CAD build for the part. Positions are in the model's coordinates, mm. Face numbers are marked on the shaded views. A direction names the side the tool comes from. Round coordinates to 2 decimals unless told otherwise and drop trailing zeros. Loops run counter-clockwise (first coordinate to the right, second up) from the corner with the lowest first, then second, coordinate; pieces in that order, holes last. Notation, with made-up numbers: M -14.75,4.5 L -2.75,4.5 A18 ccw -2.75,19.5 Z; hole C 67,85 d6. An arc over 180 degrees is marked long. Use a Markdown table: item, result. Add a question column.
(1) Band-saw the part on D-D, the plane y = 2. Write the cut outline in (x, z) (3 decimals), and give its area (3 significant figures).
(2) Band-saw the part on B-B, the plane x = 10.5. Write the cut outline in (y, z).
(3) Two-plate mould, pull along X, no slides. Class the marked faces 3, 4 and 5: released by +X, released by -X, zero draft, split by the parting line, or undercut.
(4) Wall check: L1, parallel to Z at x = 36.9, y = 12.7; L2, parallel to X at y = 27, z = 12.5; L3, parallel to Z at x = 37.85, y = 12.7. Give the ranges that are in metal, low to high.
(5) Band-saw the part on C-C, the plane z = 21.5. Write the cut outline in (x, y), and give its area (3 significant figures).
(6) Flat gauge pins, fed straight in: P1, Ø5.5, axis at y = 12.7, z = 66.075, coming from the -X side; P2, Ø6, axis at x = -15, z = 7.5, coming from the -Y side; P3, Ø3.5, axis at x = -14.5, y = 20.5, coming from the +Z side; P4, Ø7.5, axis at y = 25, z = 11, coming from the -X side. Where does each tip first touch, or does it go through?
(7) Band-saw the part on A-A, the plane y = 12.7. Give the number of separate pieces and of enclosed holes in the cut face, and give its area (3 significant figures).
(8) Which spindle directions (+Z, -Z, +X, -X, +Y, -Y) get a long thin tool onto all of the face, cutting with end or side? Do the marked faces 1 and 2. Say none if no direction does.
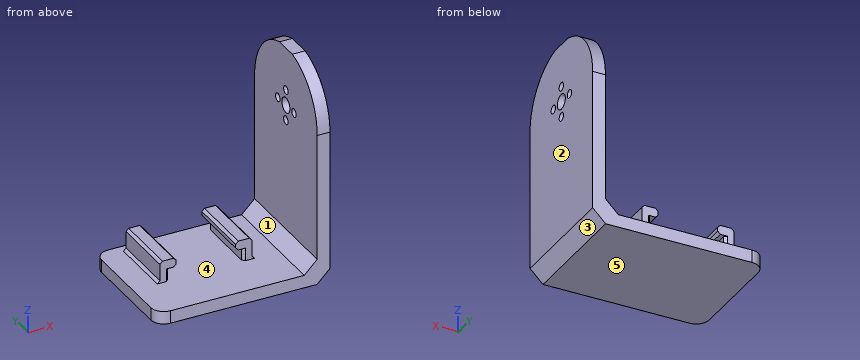
from build123d import *

# Parameters (mm, degrees)
F0_W      = 57.15
F0_H      = 21.6
F1_DEPTH  = 5
F2_W      = 57.15
F2_H      = 25.4
F3_DEPTH  = 5
F4_W      = 3.556
F4_H      = 25.4
F5_DEPTH  = 5.08
F6_W      = 6.35
F6_H      = 25.4
F7_DEPTH  = 3.556
F8_SIZE   = 1.016
F9_W      = 10.425
F9_H      = 47
F10_DEPTH = 5
F11_W     = 5
F11_H     = 47
F12_DEPTH = 78
F13_R     = 1.6478
F13_R_2   = 3
F14_DEPTH = 25.4
F16_DEPTH = 25.4
F17_R     = 5.08
F18_SIZE  = 5.08


with BuildPart() as f1:
    # F0 (on Top) → F1 (new body)
    with BuildSketch(Plane.XY):
        Rectangle(F0_W, F0_H)
    extrude(amount=F1_DEPTH)

    # F2 (on Top) → F3 (join)
    with BuildSketch(Plane.XY):
        with Locations((0, 23.5)):
            Rectangle(F2_W, F2_H)
    extrude(amount=F3_DEPTH)

    # F4 (on face) → F5 (join)
    with BuildSketch(Plane.XY.offset(5)):
        with Locations((-16.256, 20.32)):
            Rectangle(F4_W, F4_H)
        with Locations((16.256, 20.32)):
            Rectangle(F4_W, F4_H)
    extrude(amount=F5_DEPTH)

    # F6 (on face) → F7 (join)
    with BuildSketch(Plane.XY.offset(10.08)):
        with Locations((-14.859, 20.32)):
            Rectangle(F6_W, F6_H)
        with Locations((14.859, 20.32)):
            Rectangle(F6_W, F6_H)
    extrude(amount=F7_DEPTH)

    # F8
    f8_edges = [f1.edges().sort_by_distance(p)[0] for p in [
        (-11.684, 20.32, 13.636),
        (-11.684, 20.32, 10.08),
        (11.684, 20.32, 13.636),
        (11.684, 20.32, 10.08),
        (18.034, 20.32, 13.636),
        (-18.034, 20.32, 13.636),
        (18.034, 20.32, 5),
        (-18.034, 20.32, 5),
        (14.478, 33.02, 7.54),
        (-14.478, 33.02, 7.54),
        (-14.478, 7.62, 7.54),
        (14.478, 7.62, 7.54),
    ]]
    chamfer(f8_edges, length=F8_SIZE)

    # F9 (on face) → F10 (join)
    with BuildSketch(Plane.XY.offset(5)):
        with Locations((33.7875, 12.7)):
            Rectangle(F9_W, F9_H)
    extrude(amount=-F10_DEPTH)

    # F11 (on face) → F12 (join)
    with BuildSketch(Plane.XY.offset(5)):
        with Locations((36.5, 12.7)):
            Rectangle(F11_W, F11_H)
    extrude(amount=F12_DEPTH)

    # F13 (on face) → F14 (cut)
    with BuildSketch(Plane.YZ.offset(39)):
        with Locations((6.625, 60)):
            Circle(F13_R)
        with Locations((12.7, 53.925)):
            Circle(F13_R)
        with Locations((18.775, 60)):
            Circle(F13_R)
        with Locations((12.7, 66.075)):
            Circle(F13_R)
        with Locations((12.7, 60)):
            Circle(F13_R_2)
    extrude(amount=-F14_DEPTH, mode=Mode.SUBTRACT)

    # F15 (on face) → F16 (cut)
    with BuildSketch(Plane(origin=(34, 0, 0), x_dir=(0, -1, 0), z_dir=(-1, 0, 0))):
        with BuildLine():
            ThreePointArc((-36.2, 60), (-30.942298, 74.814471), (-17.521825, 83))
            Line((-17.521825, 83), (-36.2, 83))
            Line((-36.2, 83), (-36.2, 60))
        make_face()
        with BuildLine():
            Line((-17.521825, 83), (-7.878175, 83))
            ThreePointArc((-7.878175, 83), (-12.7, 83.5), (-17.521825, 83))
        make_face()
        with BuildLine():
            ThreePointArc((-7.878175, 83), (5.542298, 74.814471), (10.8, 60))
            Line((10.8, 60), (10.8, 83))
            Line((10.8, 83), (-7.878175, 83))
        make_face()
    extrude(amount=-F16_DEPTH, mode=Mode.SUBTRACT)

    # F17
    f17_edges = [f1.edges().sort_by_distance(p)[0] for p in [
        (-28.575, -10.8, 2.5),
        (-28.575, 36.2, 2.5),
    ]]
    fillet(f17_edges, radius=F17_R)

    # F18
    f18_edges = [f1.edges().sort_by_distance(p)[0] for p in [
        (34, 12.7, 5),
        (39, 12.7, 0),
    ]]
    chamfer(f18_edges, length=F18_SIZE)


solid = f1.part
Return value:
| question | item | result |
|---|---|---|
| 1 | outline | M -28.575,0 L 33.92,0 L 39,5.08 L 39,80.923 L 34,80.923 L 34,10.08 L 28.92,5 L -28.575,5 Z |
| 1 | area | 717 mm^2 |
| 2 | outline | M -10.8,0 L 36.2,0 L 36.2,5 L -10.8,5 Z |
| 3 | face 3 | released by +X |
| 3 | face 4 | undercut |
| 3 | face 5 | zero draft |
| 4 | L1 | 2.98 to 52.28, 55.57 to 57, 63 to 64.43, 67.72 to 83 |
| 4 | L2 | -18.03 to -11.68, 11.68 to 18.03, 34 to 39 |
| 4 | L3 | 3.93 to 52.28, 55.57 to 57, 63 to 64.43, 67.72 to 83 |
| 5 | outline | M 34,-10.8 L 39,-10.8 L 39,36.2 L 34,36.2 Z |
| 5 | area | 235 mm^2 |
| 6 | P1 | x = 34 |
| 6 | P2 | y = -10.8 |
| 6 | P3 | z = 13.64 |
| 6 | P4 | x = -18.03 |
| 7 | separate pieces | 4 |
| 7 | enclosed holes | 0 |
| 7 | area | 744 mm^2 |
| 8 | face 1 | +Z, +Y, -Y |
| 8 | face 2 | +Z, -Z, +X, +Y, -Y |
